Part model, mm, in its own coordinate system. Face numbers are marked on the shaded views. A direction names the side the tool comes from. Round coordinates to 2 decimals unless told otherwise and drop trailing zeros. Write each loop counter-clockwise with the first axis right and the second up, starting at its lowest first coordinate (ties: lowest second). Pieces come first, ordered by that corner, then holes. Notation, with made-up numbers: M 40,34 L 48,34 A22 cw 48,56 Z; hole C 32.5,15 d11. An arc over 180 degrees is marked long. Use a Markdown table: item, result. Add a question column.
1) Which spindle directions (+Z, -Z, +X, -X, +Y, -Y) get a long thin tool onto all of the face, cutting with end or side? Do the marked faces 5, 6 and 7. Say none if no direction does.
2) Two-plate mould, pull along X, no slides. Class the marked faces 1, 2, 3 and 4: released by +X, released by -X, zero draft, split by the parting line, or undercut.
3) Wall check: probe 1 along X at (y, z) = (-14, 5.5); probe 2 along Y at (x, z) = (3, 0); probe 3 along Y at (x, z) = (24, -6.5). Give the ranges that are in metal, low to high.
4) Slice it at C-C on y = 4.05. Write the cut outline in (x, z).
5) Slice it at B-B on z = -5. Write the cut outline in (x, y).
6) Slice it at A-A on x = 5. Write the cut outline in (y, z).
7) Slice it at D-D on y = -20.5. Write the cut outline in (x, z), plus the area to 3 significant figures.
8) Drop flat-ended pins along their axis: P1, Ø8, axis at y = -23, z = 4.5, coming from the +X side; P2, Ø5, axis at x = 5, y = 4.05, coming from the -Z side; P3, Ø5, axis at x = -19, z = -6, coming from the +Y side. Give the stop position or say it passes through.
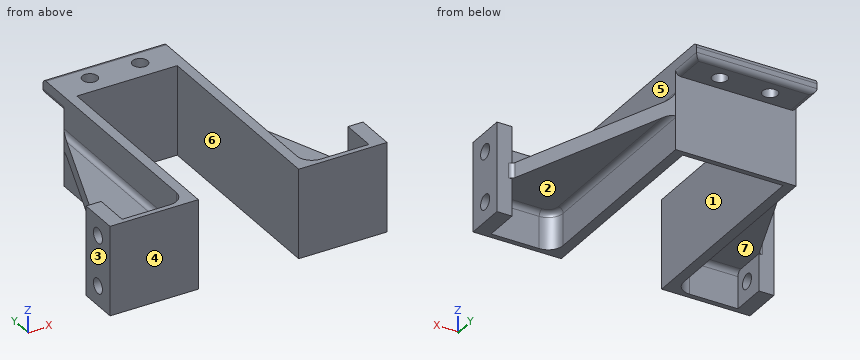
```python
from build123d import *

# Parameters (mm, degrees)
BOSS_EXTRUDE1_DEPTH = 8.9
BOSS_EXTRUDE3_START = -8.9
SKETCH5_W           = 3
SKETCH5_H           = 7
BOSS_EXTRUDE3_DEPTH = 17.8
SKETCH9_W           = 24
SKETCH9_H           = 7
SKETCH9_R           = 1.5
BOSS_EXTRUDE4_DEPTH = 3
RIB2_REACH          = 51.893
SKETCH6_WALL_W      = 137.671187546
SKETCH6_WALL_H      = 3
SKETCH7_R           = 1.5
CUT_EXTRUDE2_DEPTH  = 3
FILLET1_R           = 3
FILLET2_R           = 1


with BuildPart() as part:
    # Sketch1 → Boss-Extrude1 (new, symmetric)
    with BuildSketch(Plane.XY):
        Polygon((-10, 0), (10, 0), (10, -40.6), (27.6, -40.6), (27.6, -39.6), (12, -39.6), (12, 1), (-12, 1), (-12, -39.6), (-27.6, -39.6), (-27.6, -40.6), (-10, -40.6), align=None)
    extrude(amount=BOSS_EXTRUDE1_DEPTH, both=True)

    # Sketch5 → Boss-Extrude3 (add)
    with BuildSketch(Plane.XY.offset(BOSS_EXTRUDE3_START)):
        with Locations((-26.1, -36.1)):
            Rectangle(SKETCH5_W, SKETCH5_H)
        with Locations((26.1, -36.1)):
            Rectangle(SKETCH5_W, SKETCH5_H)
    extrude(amount=BOSS_EXTRUDE3_DEPTH)

    # Sketch9 → Boss-Extrude4 (add)
    with BuildSketch(Plane.XY.offset(8.9)):
        with Locations((0, 4.5)):
            Rectangle(SKETCH9_W, SKETCH9_H)
        with Locations((-5, 4.05)):
            Circle(SKETCH9_R, mode=Mode.SUBTRACT)
        with Locations((5, 4.05)):
            Circle(SKETCH9_R, mode=Mode.SUBTRACT)
    extrude(amount=-BOSS_EXTRUDE4_DEPTH)

    # Sketch6 wall → Rib2 (add, up to next)
    with BuildSketch(Plane(origin=(-18.3, -15.8, 0), x_dir=(0.351123441588, 0.936329177569, 0), z_dir=(-0.936329177569, 0.351123441588, 0)), mode=Mode.PRIVATE) as rib2_sk1:
        Rectangle(SKETCH6_WALL_W, SKETCH6_WALL_H)
    rib2_tool1 = extrude(rib2_sk1.sketch, amount=-RIB2_REACH, mode=Mode.PRIVATE) - part.part
    rib2 = rib2_tool1.solids().sort_by_distance((-18.3, -15.8, 0))[0]
    add(rib2)

    # Mirror3: Rib2 across plane
    add(rib2.mirror(Plane(origin=(0, 0, 0), x_dir=(0, 0, 1), z_dir=(1, 0, 0))))

    # Sketch7 → Cut-Extrude2 (cut)
    with BuildSketch(Plane.ZY.offset(27.6)):
        with Locations((-5, -36.55)):
            Circle(SKETCH7_R)
        with Locations((5, -36.55)):
            Circle(SKETCH7_R)
    cut_extrude2 = extrude(amount=-CUT_EXTRUDE2_DEPTH, mode=Mode.SUBTRACT)

    # Mirror4: Cut-Extrude2 across plane
    add(cut_extrude2.mirror(Plane(origin=(0, 0, 0), x_dir=(0, 0, 1), z_dir=(1, 0, 0))), mode=Mode.SUBTRACT)

    # Fillet1
    fillet1_edges = [part.edges().sort_by_distance(p)[0] for p in [
        (12, -39.6, -5.2),
        (-12, -39.6, 5.2),
        (12, -39.6, 5.2),
        (-12, -39.6, -5.2),
    ]]
    fillet(fillet1_edges, radius=FILLET1_R)

    # Fillet2
    fillet2_edges = [part.edges().sort_by_distance(p)[0] for p in [
        (-12, -17.8, 1.5),
        (-12, -17.8, -1.5),
        (24.6, -32.6, 0),
        (19.8, -39.6, -1.5),
        (19.8, -39.6, 1.5),
        (-19.8, -39.6, -1.5),
        (-12.878679656, -38.721320344, -1.5),
        (-19.8, -39.6, 1.5),
        (-12.878679656, -38.721320344, 1.5),
        (12, -17.8, 1.5),
        (12.878679656, -38.721320344, 1.5),
        (12, -17.8, -1.5),
        (12.878679656, -38.721320344, -1.5),
        (12, 4.5, 5.9),
        (-12, 4.5, 5.9),
        (0, 8, 5.9),
        (0, 8, 8.9),
        (-24.6, -32.6, 0),
    ]]
    fillet(fillet2_edges, radius=FILLET2_R)


solid = part.part
```
Entries:
| question | item | result |
|---|---|---|
| 1 | face 5 | +Z, +Y |
| 1 | face 6 | +Z, -Z, -Y |
| 1 | face 7 | -Z, +Y |
| 2 | face 1 | undercut |
| 2 | face 2 | undercut |
| 2 | face 3 | released by -X |
| 2 | face 4 | zero draft |
| 3 | probe 1 | x = -12 to -10, 10 to 12 |
| 3 | probe 2 | y = 0 to 1 |
| 3 | probe 3 | y = -40.6 to -39.6 |
| 4 | outline | M -12,6.9 A1 ccw -11,5.9 L -6.5,5.9 L -6.5,8.9 L -12,8.9 Z; M -3.5,5.9 L 3.5,5.9 L 3.5,8.9 L -3.5,8.9 Z; M 6.5,5.9 L 11,5.9 A1 ccw 12,6.9 L 12,8.9 L 6.5,8.9 Z |
| 5 | outline | M -27.6,-40.6 L -10,-40.6 L -10,0 L 10,0 L 10,-40.6 L 27.6,-40.6 L 27.6,-38.05 L 24.6,-38.05 L 24.6,-39.6 L 15,-39.6 A3 cw 12,-36.6 L 12,1 L -12,1 L -12,-36.6 A3 cw -15,-39.6 L -24.6,-39.6 L -24.6,-38.05 L -27.6,-38.05 Z; M -27.6,-35.05 L -24.6,-35.05 L -24.6,-32.6 L -27.6,-32.6 Z; M 24.6,-35.05 L 27.6,-35.05 L 27.6,-32.6 L 24.6,-32.6 Z |
| 6 | outline | M 0,-8.9 L 1,-8.9 L 1,5.9 L 2.55,5.9 L 2.55,8.9 L 0,8.9 Z; M 5.55,5.9 L 7,5.9 A1 ccw 8,6.9 L 8,7.9 A1 ccw 7,8.9 L 5.55,8.9 Z |
| 7 | outline | M -20.06,-1.5 L -13,-1.5 A1 cw -12,-2.5 L -12,-8.9 L -10,-8.9 L -10,8.9 L -12,8.9 L -12,2.5 A1 cw -13,1.5 L -20.06,1.5 Z; M 10,-8.9 L 12,-8.9 L 12,-2.5 A1 cw 13,-1.5 L 20.06,-1.5 L 20.06,1.5 L 13,1.5 A1 cw 12,2.5 L 12,8.9 L 10,8.9 Z |
| 7 | area | 120 mm^2 |
| 8 | P1 | stops at x = 21.99 |
| 8 | P2 | stops at z = 5.9 |
| 8 | P3 | stops at y = -39.6 |
